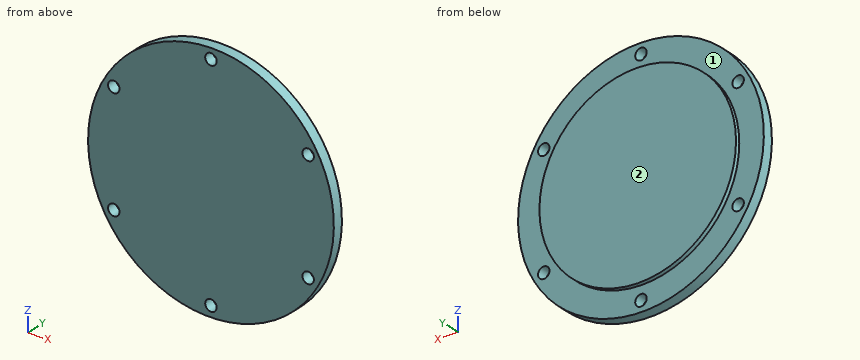
from build123d import *

# Parameters (mm, degrees)
CROQUIS1_R              = 112.5
SALIENTE_EXTRUIR1_DEPTH = 10
MATRIZC1_COUNT          = 6
CROQUIS6_R              = 90
SALIENTE_EXTRUIR2_DEPTH = 4


with BuildPart() as part:
    # Croquis1 → Saliente-Extruir1 (new body)
    with BuildSketch(Plane(origin=(0, 0, 0), x_dir=(1, 0, 0), z_dir=(0, 1, 0))):
        with Locations(Location((0, 0, 0), (0, 0, 270))):
            Circle(CROQUIS1_R)
    extrude(amount=SALIENTE_EXTRUIR1_DEPTH)

    # Croquis5 → Taladro roscado M12x1.51 (revolve, cut)
    with BuildSketch(Plane(origin=(0, 10, -102.5), x_dir=(0, 0, 1), z_dir=(1, 0, 0))):
        Polygon((0, 0), (0, 34.65451825), (5.25, 31.5), (5.25, 0), align=None)
    taladro_roscado_m12x1_51 = revolve(axis=Axis((0, 16.35, -102.5), (0, -1, 0)), mode=Mode.SUBTRACT)

    # MatrizC1: Taladro roscado M12x1.51 ×6 about axis
    matrizc1_axis = Axis((0, 0, 0.223709412), (0, 1, 0))
    for i in range(1, MATRIZC1_COUNT):
        add(taladro_roscado_m12x1_51.rotate(matrizc1_axis, i * 360 / MATRIZC1_COUNT), mode=Mode.SUBTRACT)

    # Croquis6 → Saliente-Extruir2 (add)
    with BuildSketch(Plane(origin=(0, 10, 0), x_dir=(1, 0, 0), z_dir=(0, 1, 0))):
        with Locations(Location((0, 0, 0), (0, 0, 270))):
            Circle(CROQUIS6_R)
    extrude(amount=SALIENTE_EXTRUIR2_DEPTH)


solid = part.part
Input: part model. Units: mm. Frame: model coordinates. Face numbers are marked on the shaded views. A direction names the side the tool comes from. Coordinates: 2 decimals unless noted, no trailing zeros. Loops run counter-clockwise (first coordinate to the right, second up) from the corner with the lowest first, then second, coordinate; pieces in that order, holes last.
(1) Section D-D on z = -102.5. Return the cut outline in (x, y), then the cut area to 3 significant figures.
(2) Set-up query: the marked faces 1 and 2. Return all of +Z, -Z, +X, -X, +Y, -Y with unobstructed straight access to the full face (end or side cutting, diameter ignored); none if empty.
(3) Material intervals for probe 1 along X at (y, z) = (3.5, 48); probe 2 along Z at (x, y) = (1, 4.5); probe 3 along Z at (x, y) = (-90, 7.25), sorted ascending.
(4) Section A-A on x = 0. Return the cut outline in (y, z), then the cut area to 3 significant figures.
(5) Section C-C on y = 3.5. Return the cut outline in (x, z).
(6) First-contact query: pin 1 Ø2 at (y, z) = (6.5, -14.5) entering from +X; pin 2 Ø9.5 at (x, z) = (88.96, 51.59) entering from +Y; pin 3 Ø6 at (y, z) = (5.5, 17) entering from +X; pin 4 Ø2 at (x, y) = (54.5, 5) entering from +Z. Flat tips, straight axial feed; report the tip coordinate or a pass-through.
(7) Section B-B on z = 0. Return the cut outline in (x, y), then the cut area to 3 significant figures.
Data:
1. outline: (-46.37, 0) - (-5.25, 0) - (-5.25, 10) - (-46.37, 10) - close; (5.25, 0) - (46.37, 0) - (46.37, 10) - (5.25, 10) - close
1. area: 822 mm2
2. face 1: +Y
2. face 2: +Z, -Z, +X, -X, +Y
3. probe 1: x = -101.75 to -92.8, -85.13 to 85.13, 92.8 to 101.75
3. probe 2: z = -112.5 to -107.65, -97.35 to 97.79, 108.1 to 112.5
3. probe 3: z = -67.5 to -56.28, -45.99 to 46.44, 56.73 to 67.5
4. outline: (0, -112.5) - (10, -112.5) - (10, -107.75) - (0, -107.75) - close; (0, -97.25) - (10, -97.25) - (10, -90) - (14, -90) - (14, 90) - (10, 90) - (10, 97.7) - (0, 97.7) - close; (0, 108.2) - (10, 108.2) - (10, 112.5) - (0, 112.5) - close
4. area: 2,760 mm2
5. outline: circle Ø225 at (0, 0); hole circle Ø10.5 at (-88.96, -51.14); hole circle Ø10.5 at (-88.96, 51.59); hole circle Ø10.5 at (0, -102.5); hole circle Ø10.5 at (0, 102.95); hole circle Ø10.5 at (88.96, -51.14); hole circle Ø10.5 at (88.96, 51.59)
6. pin 1: stops at x = 111.69
6. pin 2: passes through
6. pin 3: stops at x = 111.63
6. pin 4: stops at z = 98.96
7. outline: (-112.5, 0) - (112.5, 0) - (112.5, 10) - (90, 10) - (90, 14) - (-90, 14) - (-90, 10) - (-112.5, 10) - close
7. area: 2,970 mm2
